Can you work these out from the drawing? Everything is in mm from the part's minimum corner. A direction names the side the tool comes from. Coordinates: 2 decimals unless noted, no trailing zeros. Write each loop counter-clockwise with the first axis right and the second up, starting at its lowest first coordinate (ties: lowest second). Pieces come first, ordered by that corner, then holes. Notation, with made-up numbers: (-32, 6.5) -> (-14, 6.5) arc R26 cw to (-14, 28.5) -> close; hole circle Ø10 at (-7.5, 15.5). An arc over 180 degrees is marked (long way). Use a Markdown table: item, result. Add a question column.
Item 1: On a 3-axis mill with a long thin cutter (end or side, diameter ignored), from which of +Z, -Z, +X, -X, +Y, -Y can I reach the whole of each face in a straight line? I mean the marked faces 1 and 2. Say none if no direction works.
Item 2: Will this pin go through, and if not, where does the flat tip stop? pin 1 Ø3.5 at (x, z) = (64.5, 12) entering from +Y.
Item 3: Imagine slicing it at C-C, the plane y = 122.5. Write out the boundary of the cut face in (x, z), and give its area (3 significant figures).
Item 4: Imagine slicing it at B-B, the plane x = 134. Write out the boundary of the cut face in (y, z), and give its area (3 significant figures).
Item 5: Imagine slicing it at A-A, the plane y = 35.2. Write out the boundary of the cut face in (x, z), and give its area (3 significant figures).
Item 6: If I drill on line 1 along Y through (x, z) = (102, 6.25); line 2 along Y through (x, z) = (126.5, 16.5); line 3 along X through (y, z) = (120.5, 13.75), over which ranges is the centre line in solid material (lowest first)? Write a range as from..to.
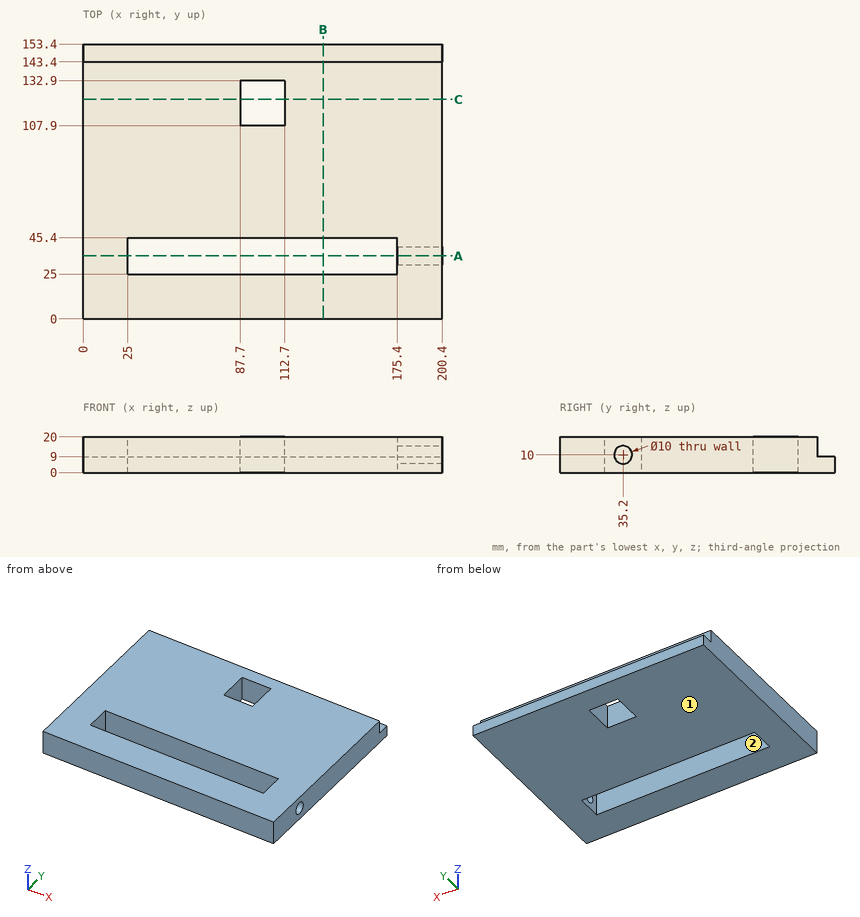
Ans:
| question | item | result |
|---|---|---|
| 1 | face 1 | -Z, +X, -X, +Y, -Y |
| 1 | face 2 | +Z, -Z |
| 2 | pin 1 | stops at y = 143.4 |
| 3 | outline | (0, 0) -> (87.7, 0) -> (87.7, 20) -> (0, 20) -> close; (112.7, 0) -> (200.4, 0) -> (200.4, 20) -> (112.7, 20) -> close |
| 3 | area | 3,510 mm^2 |
| 4 | outline | (0, 0) -> (25, 0) -> (25, 20) -> (0, 20) -> close; (45.4, 0) -> (153.4, 0) -> (153.4, 9) -> (143.4, 9) -> (143.4, 20) -> (45.4, 20) -> close |
| 4 | area | 2,550 mm^2 |
| 5 | outline | (0, 0) -> (25, 0) -> (25, 20) -> (0, 20) -> close; (175.4, 0) -> (200.4, 0) -> (200.4, 5) -> (175.4, 5) -> close; (175.4, 15) -> (200.4, 15) -> (200.4, 20) -> (175.4, 20) -> close |
| 5 | area | 750 mm^2 |
| 6 | line 1 | y = 0..25, 45.4..107.9, 132.9..153.4 |
| 6 | line 2 | y = 0..25, 45.4..143.4 |
| 6 | line 3 | x = 0..87.7, 112.7..200.4 |
